from build123d import *

# Parameters (mm, degrees)
F1_DEPTH       = 3.175
F2_D           = 3.7973
F2_CSINK_D     = 7.7978
F2_CSINK_ANGLE = 82


# Not quite as in the source:
# - a feature of the source that left no trace in its solid (it failed there, or was rolled back) is left out


with BuildPart() as f1:
    # F0 (on Top) → F1 (new body)
    with BuildSketch(Plane.XY):
        with BuildLine():
            Line((81.75625, 38.1), (-81.75625, 38.1))
            ThreePointArc((-81.75625, 38.1), (-82.3175160076, 37.8675160076), (-82.55, 37.30625))
            Line((-82.55, 37.30625), (-82.55, -37.30625))
            ThreePointArc((-82.55, -37.30625), (-82.3175160076, -37.8675160076), (-81.75625, -38.1))
            Line((-81.75625, -38.1), (81.75625, -38.1))
            ThreePointArc((81.75625, -38.1), (82.3175160076, -37.8675160076), (82.55, -37.30625))
            Line((82.55, -37.30625), (82.55, 37.30625))
            ThreePointArc((82.55, 37.30625), (82.3175160076, 37.8675160076), (81.75625, 38.1))
        make_face()
    extrude(amount=F1_DEPTH)

    # F2 (through all)
    with Locations(Plane(origin=(0, 0, 0), x_dir=(1, 0, 0), z_dir=(0, 0, -1))):
        with Locations((49.2125, 33.3375), (71.4375, 33.3375), (60.325, -12.7), (0, -12.7), (-60.325, -12.7)):
            CounterSinkHole(F2_D / 2, F2_CSINK_D / 2, counter_sink_angle=F2_CSINK_ANGLE)


solid = f1.part
Input: part model. Units: mm. Frame: model coordinates. Coordinates: 2 decimals unless noted, no trailing zeros. Loops run counter-clockwise (first coordinate to the right, second up) from the corner with the lowest first, then second, coordinate; pieces in that order, holes last. Notation, with made-up numbers: (53, 35.25) -> (94, 35.25) arc R27 cw to (94, 74.25) -> close; hole circle Ø8 at (19, 82). An arc over 180 degrees is marked (long way). Write each question's results on one line, items separated by ' | '. Start each with the question number.
Q1. Ray query, line 1 (X direction, y = 12.7, z = 2.8); line 2 (Y direction, x = 74.5, z = 0.65); line 3 (Y direction, x = 1, z = 3). Return the intervals inside material, ascending. Write a range as from..to.
Q2. Pin query (flat end, axial travel): pin 1 (6 mm diameter, centred on x = 60.325, y = 12.7, fed in from -Z). Return the tip coordinate at first contact, or that it passes through.
Q3. Pull-direction query (Y, two-part tool) for faces 1 (the cylindrical face through (47.4, -33.9, 2.7)), 2 (the cylindrical face through (-58.926, 11.417, 2.744)), 3 (the flat face through (-1, -38.1, 2)), 4 (the flat face through (-1, 1, 3.175)); classes: released by +Y, released by -Y, zero draft, split by the parting line, or undercut.
Q4. Section A-A, the plane y = 12.7. Return the cut outline in (x, z) (3 decimals).
Q5. Section B-B, the plane x = 0. Return the cut outline in (y, z) (3 decimals).
Found:
1) line 1: -82.55..-62.22, -58.43..-1.9, 1.9..58.43, 62.22..82.55 | line 2: -38.1..-34.65, -32.02..38.1 | line 3: -38.1..11.09, 14.31..38.1
2) pin 1: z = 1.03
3) face 1: undercut | face 2: undercut | face 3: released by -Y | face 4: zero draft
4) outline: (-82.55, 0) -> (-64.224, 0) -> (-62.224, 2.301) -> (-62.224, 3.175) -> (-82.55, 3.175) -> close; (-58.426, 2.301) -> (-56.426, 0) -> (-3.899, 0) -> (-1.899, 2.301) -> (-1.899, 3.175) -> (-58.426, 3.175) -> close; (1.899, 2.301) -> (3.899, 0) -> (56.426, 0) -> (58.426, 2.301) -> (58.426, 3.175) -> (1.899, 3.175) -> close; (62.224, 2.301) -> (64.224, 0) -> (82.55, 0) -> (82.55, 3.175) -> (62.224, 3.175) -> close
5) outline: (-38.1, 0) -> (8.801, 0) -> (10.801, 2.301) -> (10.801, 3.175) -> (-38.1, 3.175) -> close; (14.599, 2.301) -> (16.599, 0) -> (38.1, 0) -> (38.1, 3.175) -> (14.599, 3.175) -> close
